Could you check a few things on this drawing? It's one solid part, dimensions in mm from its lowest x, y, z. A direction names the side the tool comes from. Give positions to 0.01 mm unless a question says otherwise; leave off trailing zeros. Order: outer loops, then holes, each group sorted by start corner. A loop starts at its lowest first (then second) coordinate and runs counter-clockwise, first axis right, second up.
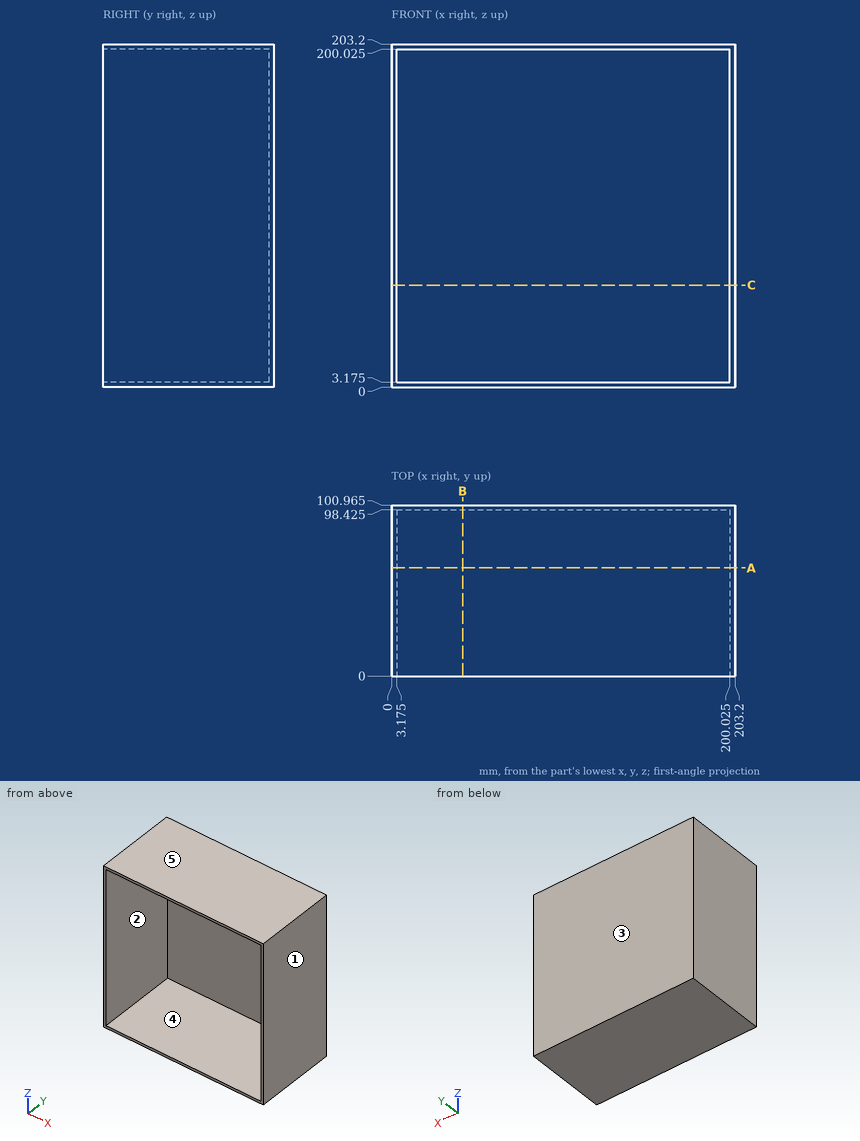
Item 1: Imagine slicing it at B-B on x = 42. List the corners of the cut face in (y, z) for me (3 decimals), then the cut area to 3 significant figures.
Findings:
outline: (0, 0) - (100.965, 0) - (100.965, 203.2) - (0, 203.2) - (0, 200.025) - (98.425, 200.025) - (98.425, 3.175) - (0, 3.175) - close
area: 1,140 mm2
Item 2: Imagine slicing it at C-C on z = 60.5. List the corners of the cut face in (x, y) for me (3 decimals), then the cut area to 3 significant figures.
Findings:
outline: (0, 0) - (3.175, 0) - (3.175, 98.425) - (200.025, 98.425) - (200.025, 0) - (203.2, 0) - (203.2, 100.965) - (0, 100.965) - close
area: 1,140 mm2
Item 3: We'd pull the mould along Z, two halves only. Please class the marked faces 3, 4 and 5: +Z half, -Z half, draft (parallel to the pull), parting line (faces both ways), or undercut.
Findings:
face 3: draft
face 4: undercut
face 5: +Z half
Item 4: Imagine slicing it at A-A on y = 64. List the corners of the cut face in (x, z) for me (3 decimals).
Findings:
outline: (0, 0) - (203.2, 0) - (203.2, 203.2) - (0, 203.2) - close; hole (3.175, 3.175) - (200.025, 3.175) - (200.025, 200.025) - (3.175, 200.025) - close
Item 5: For the marked faces 1 and 2, which set-ups out of +Z, -Z, +X, -X, +Y, -Y let a thin tool reach every point of the face, with its end or its side?
Findings:
face 1: +Z, -Z, +X, +Y, -Y
face 2: -Y
Item 6: Please list where these lines run through material, in increasing order: line 1 along X through (y, z) = (53, 195.5) (3 decimals); line 2 along Y through (x, z) = (12, 156) (3 decimals).
Findings:
line 1: x = 0 to 3.175, 200.025 to 203.2
line 2: y = 98.425 to 100.965
